Input: dimensioned drawing with shaded views. Units: mm. Origin: part minimum x, y, z. A direction names the side the tool comes from. Coordinates: 2 decimals unless noted, no trailing zeros. Loops run counter-clockwise (first coordinate to the right, second up) from the corner with the lowest first, then second, coordinate; pieces in that order, holes last.
Item 1: Section A-A on y = 5. Return loops of the section in (x, z).
Item 2: Section C-C on z = 6. Return loops of the section in (x, y), and give its area (3 significant figures).
Item 3: Section B-B on x = 14.25. Return loops of the section in (y, z) (1 decimal), and give its area (3 significant figures).
Item 4: Section D-D on x = 2.5. Return loops of the section in (y, z) (1 decimal), and give its area (3 significant figures).
Item 5: Ray query, line 1 along X through (y, z) = (15.75, 8.5) (1 decimal); line 2 along Z through (x, y) = (6.25, 19.25); line 3 along Y through (x, z) = (8, 3.5) (1 decimal). Return the intervals inside material, ascending.
Item 6: Reachability of the marked faces 4, 5 and 6 from +Z, -Z, +X, -X, +Y, -Y: full face, straight path, thin tool, end or side. Return the list, or none.
Item 7: Contact query for flat-ended pins moving along their axis: P1, Ø8, axis at y = 7.5, z = 12, coming from the +X side; P2, Ø2, axis at x = 11.5, z = 15, coming from the +Y side; P3, Ø2.5, axis at y = 18.5, z = 19, coming from the -X side (1 decimal); P4, Ø3.5, axis at y = 3, z = 19, coming from the -X side. Output: stop coordinate, or through.
Item 8: Pull-direction query (X, two-part tool) for the marked faces 1, 2 and 3; classes: released by +X, released by -X, zero draft, split by the parting line, or undercut.
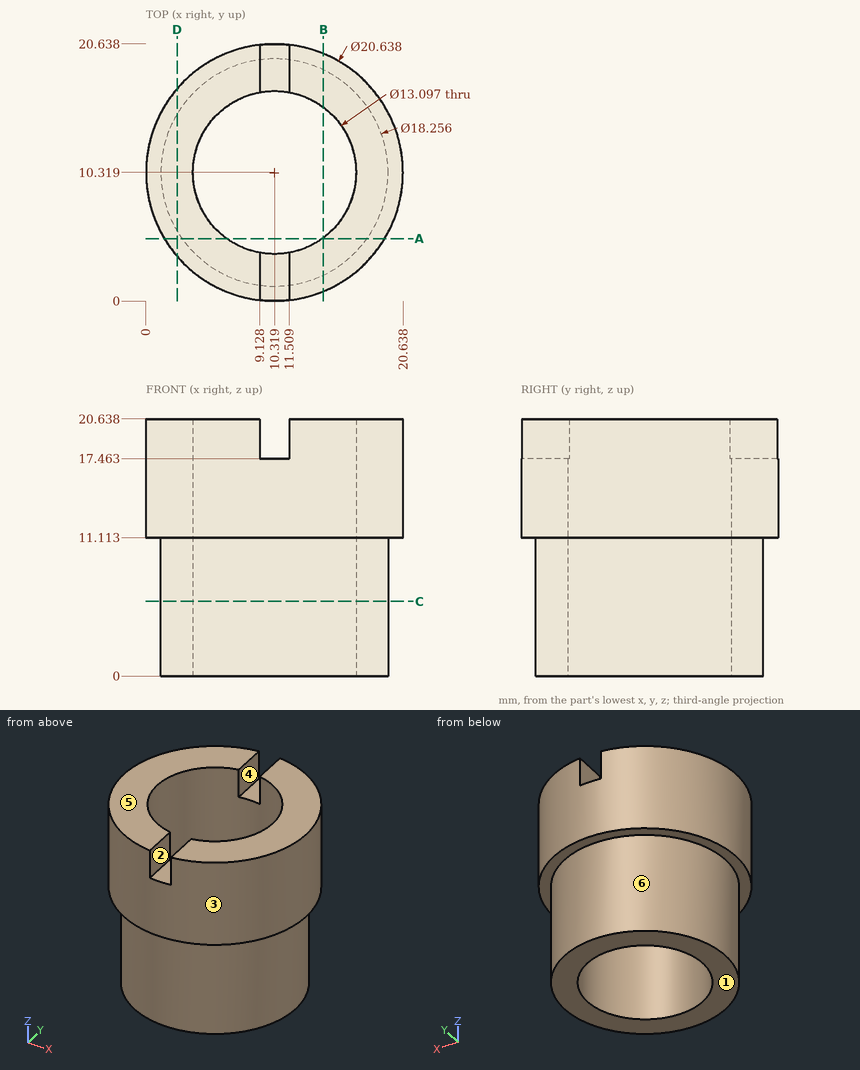
Results found:
1. outline: (1.48, 11.11) - (2.9, 11.11) - (2.9, 0) - (6.5, 0) - (6.5, 20.64) - (1.48, 20.64) - close; (14.14, 0) - (17.74, 0) - (17.74, 11.11) - (19.16, 11.11) - (19.16, 20.64) - (14.14, 20.64) - close
2. outline: circle Ø18.26 at (10.32, 10.32); hole circle Ø13.1 at (10.32, 10.32)
2. area: 127 mm2
3. outline: (0.8, 11.1) - (2.1, 11.1) - (2.1, 0) - (5.1, 0) - (5.1, 20.6) - (0.8, 20.6) - close; (15.6, 0) - (18.6, 0) - (18.6, 11.1) - (19.9, 11.1) - (19.9, 20.6) - (15.6, 20.6) - close
3. area: 149 mm2
4. outline: (3.6, 11.1) - (5.6, 11.1) - (5.6, 0) - (15, 0) - (15, 11.1) - (17.1, 11.1) - (17.1, 20.6) - (3.6, 20.6) - close
4. area: 233 mm2
5. line 1: x = 3 to 6.7, 14 to 17.7
5. line 2: z = 11.11 to 20.64
5. line 3: y = 1.5 to 4.2, 16.4 to 19.1
6. face 4: +Z, +Y, -Y
6. face 5: +Z, +X, -X, +Y, -Y
6. face 6: -Z
7. P1: stops at x = 20.64
7. P2: stops at y = 20.64
7. P3: stops at x = 2.7
7. P4: stops at x = 1.63
8. face 1: zero draft
8. face 2: undercut
8. face 3: split by the parting line
